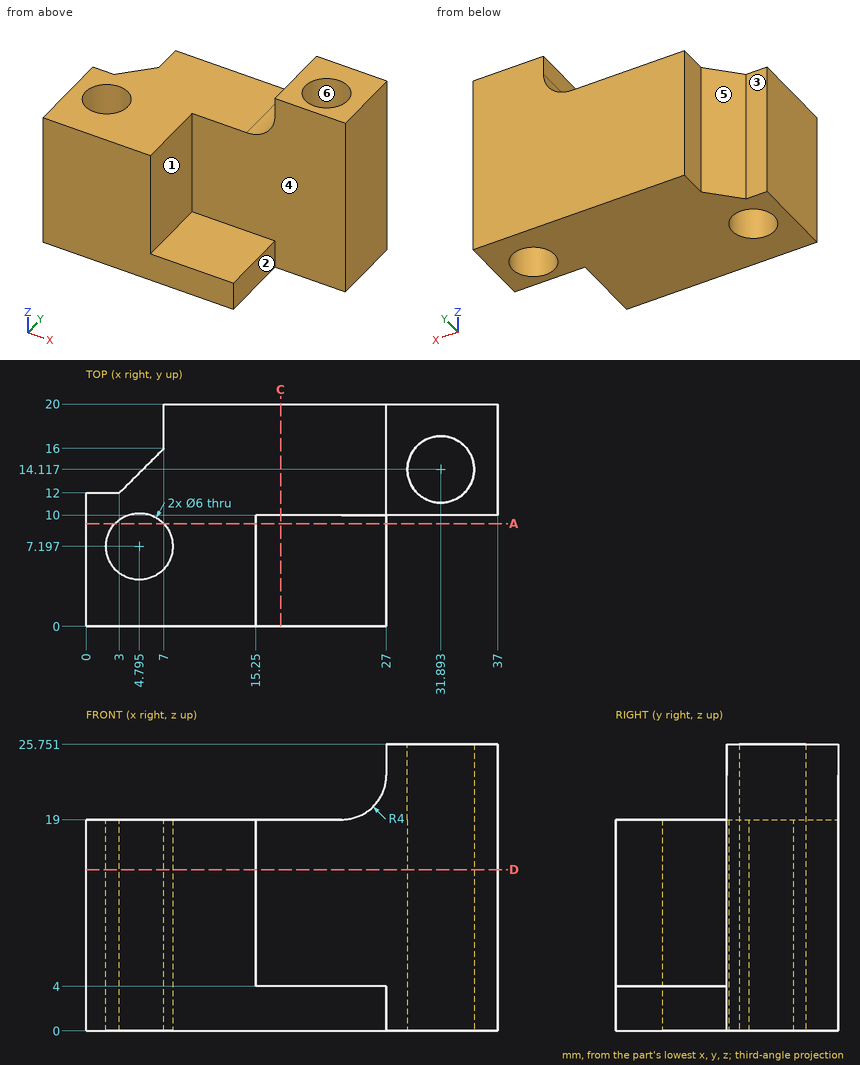
Source: three-view drawing plus pictorial views. Frame: mm from the lowest corner of the part. A direction names the side the tool comes from. Give positions to 0.01 mm unless a question says otherwise; leave off trailing zeros. Order: outer loops, then holes, each group sorted by start corner. A loop starts at its lowest first (then second) coordinate and runs counter-clockwise, first axis right, second up. Notation, with made-up numbers: M 65,25.5 L 93,25.5 A20 ccw 93,44.5 Z; hole C 75,19.5 d8. An arc over 180 degrees is marked long. One line per question, with ' | ' between items.
1) Section C-C on x = 17.5. Output: boundary loops of the cut face in (y, z).
Filled in:
outline: M 0,0 L 20,0 L 20,19 L 10,19 L 10,4 L 0,4 Z
2) Ray query, L1, parallel to Z at x = 8, y = 6; L2, parallel to X at y = 2, z = 12.5; L3, parallel to Y at x = 23, z = 18. Return the intervals inside material, ascending.
Filled in:
L1: z = 0 to 19 | L2: x = 0 to 15.25 | L3: y = 10 to 20
3) Section D-D on z = 14.5. State how many separate pieces and enclosed holes the cut face has, and give its area (3 significant figures).
Filled in:
separate pieces: 1 | enclosed holes: 2 | area: 418 mm2
4) Draft query along X for the marked faces 4, 5 and 6. Return one class per face: pulls with the +X half, pulls with the -X half, needs draft (parallel to the pull), parting line crosses it, or undercut.
Filled in:
face 4: needs draft | face 5: pulls with the -X half | face 6: undercut
5) Contact query for flat-ended pins moving along their axis: P1, Ø3, axis at y = 9.5, z = 22.5, coming from the +X side; P2, Ø2, axis at y = 14, z = 23.5, coming from the -X side; P3, Ø3, axis at y = 5, z = 2, coming from the +X side; P4, Ø4.5, axis at y = 18.5, z = 5.5, coming from the -X side. Output: stop coordinate, or through.
Filled in:
P1: stops at x = 37 | P2: stops at x = 26.97 | P3: stops at x = 27 | P4: stops at x = 7
6) Access query for the marked faces 1, 2 and 3. Directions: +Z, -Z, +X, -X, +Y, -Y. A direction counts if a zero-diameter tool reaches every point of the face in a straight line with its end or side. Return the directions, or none.
Filled in:
face 1: +Z, +X, -Y | face 2: +Z, -Z, +X, -Y | face 3: +Z, -Z, -X, +Y
7) Section A-A on y = 9.25. Output: boundary loops of the cut face in (x, z).
Filled in:
outline: M 0,0 L 2.61,0 L 2.61,19 L 0,19 Z; M 6.98,0 L 27,0 L 27,4 L 15.25,4 L 15.25,19 L 6.98,19 Z
